The listing builds one solid part. Answer for the finished solid, in the listing's coordinates (mm). Face numbers are marked on the shaded views. A direction names the side the tool comes from. Round coordinates to 2 decimals unless told otherwise and drop trailing zeros. Order: outer loops, then holes, each group sorted by start corner. A loop starts at its lowest first (then second) coordinate and runs counter-clockwise, first axis right, second up. Notation, with made-up numbers: (40, 59.25) - (50, 59.25) arc R24 ccw to (50, 86.25) - close; hole circle Ø11 at (77, 74). An arc over 180 degrees is marked (long way). Use CSV: the item, a comma, the result in double quotes. Start each with the question number.
Item 1: Find section D-D, the plane x = 11. Give the vertices of the cut face in (y, z).
Item 2: Straight lines are drawn through the part: line 1 along Z through (x, y) = (27, -2); line 2 along X through (y, z) = (-6, 32); line 3 along Z through (x, y) = (-4.5, -17). For each, find the intervals that lie inside material, in ascending order. Write a range as [from, to].
Item 3: Flat-ended cylindrical pins translate along their axes: P1, Ø3, axis at y = 14, z = 33, coming from the -X side (3 decimals); P2, Ø1.5, axis at x = -22, y = -9, coming from the +Z side; P3, Ø12, axis at x = 16.5, z = 31.5, coming from the +Y side. Find the tip coordinate at first contact, or state that the pin passes through.
Item 4: Determine the mould class of the marked faces 6, 7 and 8 for opening direction X: +X half, -X half, draft (parallel to the pull), parting line (faces both ways), or undercut.
Item 5: For the marked faces 1, 2, 3, 4 and 5, determine the directions among +Z, -Z, +X, -X, +Y, -Y from which every point of the face is accessible in a straight line to the end or side of a thin tool.
Item 6: Find section A-A, the plane z = 8. Give the vertices of the cut face in (x, y).
Item 7: Find section B-B, the plane y = 8. Give the vertices of the cut face in (x, z).
Item 8: Find section C-C, the plane z = 28. Give the vertices of the cut face in (x, y).
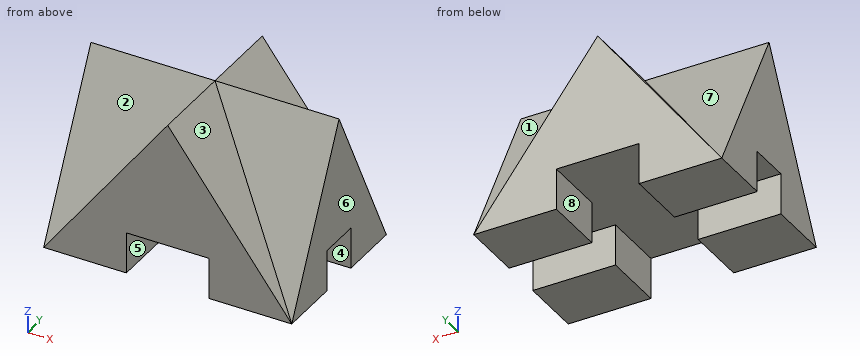
```python
from build123d import *

# Parameters (mm, degrees)
F1_DEPTH = 20
F3_DEPTH = 30
F4_W     = 20
F4_H     = 10
F5_DEPTH = 40
F6_W     = 10
F6_H     = 10
F7_DEPTH = 64.9


with BuildPart() as f1:
    # F0 (on Front) → F1 (new body, symmetric)
    with BuildSketch(Plane.XZ):
        Polygon((0, 40), (-30, 0), (30, 0), align=None)
    extrude(amount=F1_DEPTH, both=True)

    # F2 (on Right) → F3 (join, symmetric)
    with BuildSketch(Plane.YZ):
        Polygon((20, 0), (0, 40), (-20, 0), align=None)
    extrude(amount=F3_DEPTH, both=True)

    # F4 (on face) → F5 (cut, through all)
    with BuildSketch(Plane.XZ.offset(20)):
        with Locations((0, 5)):
            Rectangle(F4_W, F4_H)
    extrude(amount=-F5_DEPTH, mode=Mode.SUBTRACT)

    # F6 (on face) → F7 (cut)
    with BuildSketch(Plane.YZ.offset(30)):
        with Locations((0, 5)):
            Rectangle(F6_W, F6_H)
    extrude(amount=-F7_DEPTH, mode=Mode.SUBTRACT)


solid = f1.part
```
Worked out:
1,outline,"(-20, 0) - (-5, 0) - (-5, 10) - (5, 10) - (5, 0) - (20, 0) - (20, 25.33) - (7.33, 25.33) - (0, 40) - (-7.33, 25.33) - (-20, 25.33) - close"
2,line 1,"z = [10, 36]"
2,line 2,"x = [-6, 6]"
2,line 3,"z = [10, 34]"
3,P1,"stops at x = -6.375"
3,P2,"stops at z = 23.5"
3,P3,"stops at y = 7.25"
4,face 6,"+X half"
4,face 7,"draft"
4,face 8,"undercut"
5,face 1,"+Z, +X, +Y"
5,face 2,"+Z, -X, -Y"
5,face 3,"+Z, +X, -Y"
5,face 4,"-Z, +X, -X"
5,face 5,"-Z, +Y, -Y"
6,outline,"(-30, -16) - (-24, -16) - (-24, -20) - (-10, -20) - (-10, -5) - (-30, -5) - close; (-30, 5) - (-10, 5) - (-10, 20) - (-24, 20) - (-24, 16) - (-30, 16) - close; (10, -20) - (24, -20) - (24, -16) - (30, -16) - (30, -5) - (10, -5) - close; (10, 5) - (30, 5) - (30, 16) - (24, 16) - (24, 20) - (10, 20) - close"
7,outline,"(-30, 0) - (-10, 0) - (-10, 10) - (10, 10) - (10, 0) - (30, 0) - (30, 24) - (12, 24) - (0, 40) - (-12, 24) - (-30, 24) - close"
8,outline,"(-30, -6) - (-9, -6) - (-9, -20) - (9, -20) - (9, -6) - (30, -6) - (30, 6) - (9, 6) - (9, 20) - (-9, 20) - (-9, 6) - (-30, 6) - close"
